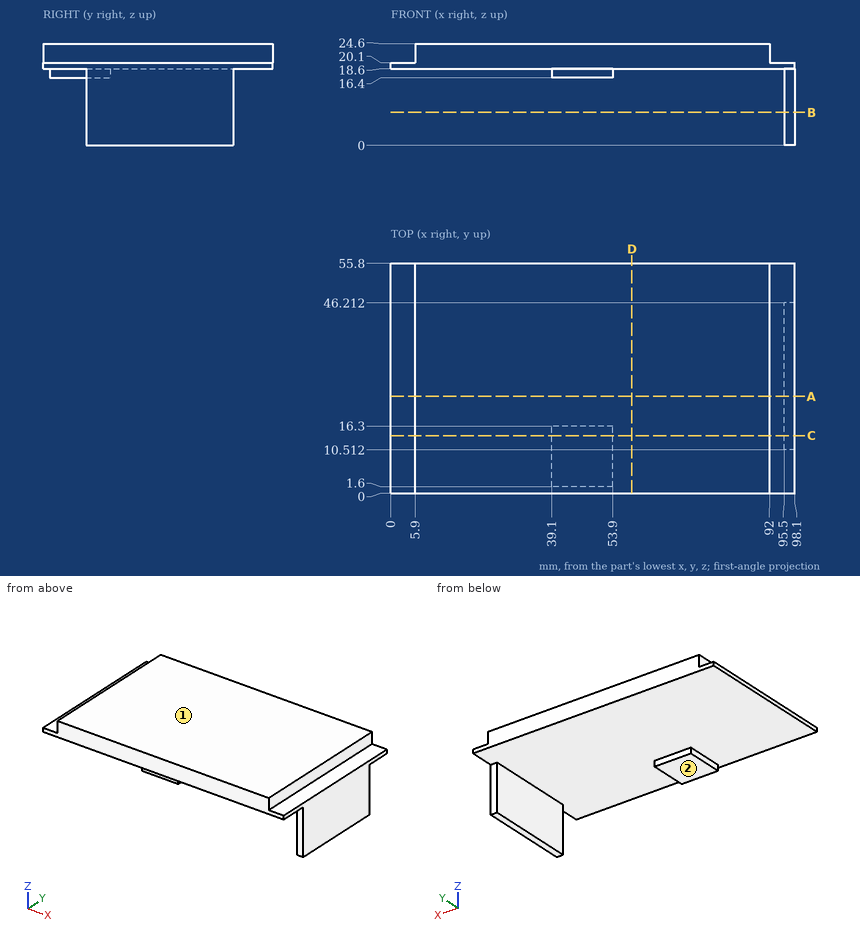
Geometry check sheet. Reference: drawing and pictorial views, mm from the part's lowest x, y, z. A direction names the side the tool comes from. Round coordinates to 2 decimals unless told otherwise and drop trailing zeros. Order: outer loops, then holes, each group sorted by start corner. A loop starts at its lowest first (then second) coordinate and runs counter-clockwise, first axis right, second up.
Q1. Cross-section at D-D, the plane x = 58.5. Enter the section's corners in (y, z), plus the area to 3 significant figures.
Filled sheet:
outline: (0, 18.6) - (55.8, 18.6) - (55.8, 24.6) - (0, 24.6) - close
area: 335 mm2
Q2. Set-up check for the marked faces 1 and 2: record each of +Z, -Z, +X, -X, +Y, -Y from which the full face is reachable in a straight line by a thin tool's end or side.
Filled sheet:
face 1: +Z, +X, -X, +Y, -Y
face 2: -Z, -X, +Y, -Y
Q3. Cross-section at B-B, the plane z = 8. Enter the section's corners in (x, y).
Filled sheet:
outline: (95.5, 10.51) - (98.1, 10.51) - (98.1, 46.21) - (95.5, 46.21) - close
Q4. Scan lines: L1, parallel to X at y = 4.5, z = 18.5; L2, parallel to X at y = 38, z = 2; L3, parallel to Z at x = 51, y = 49. Record each from-to range of solid material in increasing order.
Filled sheet:
L1: x = 39.1 to 53.9
L2: x = 95.5 to 98.1
L3: z = 18.6 to 24.6
Q5. Cross-section at C-C, the plane y = 14. Enter the section's corners in (x, z).
Filled sheet:
outline: (0, 18.6) - (39.1, 18.6) - (39.1, 16.4) - (53.9, 16.4) - (53.9, 18.6) - (95.5, 18.6) - (95.5, 0) - (98.1, 0) - (98.1, 20.1) - (92, 20.1) - (92, 24.6) - (5.9, 24.6) - (5.9, 20.1) - (0, 20.1) - close
Q6. Cross-section at A-A, the plane y = 23.5. Enter the section's corners in (x, z).
Filled sheet:
outline: (0, 18.6) - (95.5, 18.6) - (95.5, 0) - (98.1, 0) - (98.1, 20.1) - (92, 20.1) - (92, 24.6) - (5.9, 24.6) - (5.9, 20.1) - (0, 20.1) - close
Q7. Depth check by flat-ended pin: P1, Ø5, axis at y = 10, z = 21, coming from the +X side; P2, Ø6.5, axis at x = 95.5, y = 22.5, coming from the +Z side; P3, Ø1.1, axis at y = 8.5, z = 17, coming from the -X side; P4, Ø1.5, axis at y = 38, z = 21, coming from the +X side. Enter the tip coordinate at first touch or a pass-through.
Filled sheet:
P1: stops at x = 98.1
P2: stops at z = 20.1
P3: stops at x = 39.1
P4: stops at x = 92
